Part model, mm, in its own coordinate system. A direction names the side the tool comes from. Round coordinates to 2 decimals unless told otherwise and drop trailing zeros. Write each loop counter-clockwise with the first axis right and the second up, starting at its lowest first coordinate (ties: lowest second). Pieces come first, ordered by that corner, then holes.
1) Flat gauge pins, fed straight in: pin 1 (3 mm diameter, centred on x = -3, y = 7, fed in from -Z); pin 2 (4 mm diameter, centred on x = 3.5, y = 10.5, fed in from +Z); pin 3 (2 mm diameter, centred on y = 8.5, z = 3.5, fed in from +X). Where does each tip first touch, or does it go through?
2) Saw through at A-A on z = 0. Write the cut outline in (x, y).
3) Pull direction X, two halves, no side cores. Call faces 1 (the flat face through (1, 25, 3)), 2 (the cylindrical face through (-2.103, 12.332, -6.677)), 3 (the cylindrical face through (-0.9, 18.84, -2.86)): +X half, -X half, draft (parallel to the pull), parting line (faces both ways), or undercut.
4) Saw through at D-D on y = 6.25. Write the cut outline in (x, z), and give its area (3 significant figures).
5) Saw through at C-C on y = 22.25. Write the cut outline in (x, z), and give its area (3 significant figures).
6) Saw through at B-B on x = 0. Write the cut outline in (y, z).
7) Which spindle directions (+Z, -Z, +X, -X, +Y, -Y) get a long thin tool onto all of the face, cutting with end or side? Do faces 4 (the cylindrical face through (1.532, 6.338, -3.695)), 5 (the flat face through (-3, 0, -3)), 6 (the cylindrical face through (-1.65, 6.32, 5.35)). Say none if no direction does.
8) Drill centre lines: L1, parallel to Y at x = 0, z = 4.8; L2, parallel to Y at x = 0, z = 3.75; L3, parallel to X at y = 18.75, z = 3.75. Where is each one in solid material? Low to high.
```python
from build123d import *

# Parameters (mm, degrees)
CHAMFER1_SIZE          = 0.5
M4_TAPPED_HOLE1_REACH  = 31.496
M4_TAPPED_HOLE1_BORE_R = 1.65


with BuildPart() as part:
    # Sketch2 → Revolve1 (revolve)
    with BuildSketch(Plane(origin=(0, 0, 0), x_dir=(0, 0, -1), z_dir=(1, 0, 0))):
        Polygon((4, 0), (4, 12.5), (3, 12.5), (3, 25), (7, 25), (7, 0), align=None)
    revolve(axis=Axis((0, 0, 0), (0, 1, 0)))

    # Chamfer1
    chamfer1_edges = [part.edges().sort_by_distance(p)[0] for p in [
        (0, 0, 7),
        (0, 25, 7),
    ]]
    chamfer(chamfer1_edges, length=CHAMFER1_SIZE)

    # M4 Tapped Hole1 bore → M4 Tapped Hole1 (cut, up to next)
    with BuildSketch(Plane.XY.offset(7), mode=Mode.PRIVATE) as m4_tapped_hole1_sk1:
        with Locations((0, 18.75)):
            Circle(M4_TAPPED_HOLE1_BORE_R)
    m4_tapped_hole1_tool1 = extrude(m4_tapped_hole1_sk1.sketch, amount=-M4_TAPPED_HOLE1_REACH, mode=Mode.PRIVATE) & part.part
    # M4 Tapped Hole1 bore → M4 Tapped Hole1 (cut, up to next)
    with BuildSketch(Plane.XY.offset(7), mode=Mode.PRIVATE) as m4_tapped_hole1_sk2:
        with Locations((0, 6.25)):
            Circle(M4_TAPPED_HOLE1_BORE_R)
    m4_tapped_hole1_tool2 = extrude(m4_tapped_hole1_sk2.sketch, amount=-M4_TAPPED_HOLE1_REACH, mode=Mode.PRIVATE) & part.part
    add(m4_tapped_hole1_tool1.solids().sort_by_distance((0, 18.75, 7))[0], mode=Mode.SUBTRACT)
    add(m4_tapped_hole1_tool2.solids().sort_by_distance((0, 6.25, 7))[0], mode=Mode.SUBTRACT)


solid = part.part
```
Completed:
1. pin 1: stops at z = -6.84
1. pin 2: stops at z = 6.84
1. pin 3: stops at x = 6.54
2. outline: (-7, 0.5) - (-6.5, 0) - (-4, 0) - (-4, 12.5) - (-3, 12.5) - (-3, 25) - (-6.5, 25) - (-7, 24.5) - close; (3, 12.5) - (4, 12.5) - (4, 0) - (6.5, 0) - (7, 0.5) - (7, 24.5) - (6.5, 25) - (3, 25) - close
3. face 1: draft
3. face 2: parting line
3. face 3: undercut
4. outline: (-1.65, 3.64) - (-1.65, 6.8) arc R7 ccw (long way) to (1.65, 6.8) - (1.65, 3.64) arc R4 cw (long way) to start
4. area: 93.6 mm2
5. outline: circle Ø14 at (0, 0); hole circle Ø6 at (0, 0)
5. area: 126 mm2
6. outline: (0, -6.5) - (0.5, -7) - (24.5, -7) - (25, -6.5) - (25, -3) - (12.5, -3) - (12.5, -4) - (0, -4) - close; (0, 4) - (4.6, 4) - (4.6, 7) - (0.5, 7) - (0, 6.5) - close; (7.9, 4) - (12.5, 4) - (12.5, 3) - (17.1, 3) - (17.1, 7) - (7.9, 7) - close; (20.4, 3) - (25, 3) - (25, 6.5) - (24.5, 7) - (20.4, 7) - close
7. face 4: -Y
7. face 5: +Z, -Z, +X, -X, -Y
7. face 6: +Z
8. L1: y = 0 to 4.6, 7.9 to 17.1, 20.4 to 25
8. L2: y = 12.5 to 17.1, 20.4 to 25
8. L3: x = -5.91 to -1.65, 1.65 to 5.91
